Autodesk Inventor part; units mm, degrees
ref_plane "YZ Plane" through (0, 0, 0) normal (1, 0, 0) x (0, 1, 0)
ref_plane "XZ Plane" through (0, 0, 0) normal (0, 1, 0) x (-1, 0, 0)
ref_plane "XY Plane" through (0, 0, 0) normal (0, 0, 1) x (1, 0, 0)
sketch "Boceto1" plane through (0, 0, 0) normal (0, 1, 0) x (-1, 0, 0)
  line L0 (0, 0) -> (0, -8.25)
  line L1 (0, -8.25) -> (3, -8.25)
  line L2 (3, -8.25) -> (3, -16.5)
  line L3 (3, -16.5) -> (0, -16.5)
  line L4 (0, -16.5) -> (0, -24.75)
  line L5 (0, -24.75) -> (3, -24.75)
  line L6 (3, -24.75) -> (3, -33)
  line L7 (3, -33) -> (20, -33)
  line L8 (20, 0) -> (0, 0)
  line L9 (20, -28) -> (8, -28)
  line L10 (8, -28) -> (8, -5)
  line L11 (8, -5) -> (20, -5)
  line L12 (20, -33) -> (20, -28)
  line L13 (20, -5) -> (20, 0)
  dimension "d0" = 8.25
  dimension "d1" = 3
  dimension "d3" = 8.25
extrude "Extrusión1" add sketch "Boceto1" along normal blind 3
sketch "Boceto2" plane through (0, 0, 0) normal (0, -1, 0) x (1, 0, 0)
  line L0 (-8, -28) -> (-8, -5)
  line L1 (-8, -5) -> (-8, -28)
  line L2 (-8, -28) -> (-6, -28)
  line L3 (-6, -28) -> (-6, -5)
  line L4 (-6, -5) -> (-8, -5)
  line L5 (-20, 0) -> (-20, -5)
  line L6 (-20, -5) -> (-18, -5)
  line L7 (-18, -5) -> (-18, 0)
  line L8 (-18, 0) -> (-20, 0)
  line L9 (-20, -33) -> (-20, -28)
  line L10 (-20, -28) -> (-18, -28)
  line L11 (-18, -28) -> (-18, -33)
  line L12 (-18, -33) -> (-20, -33)
extrude "Extrusión2" cut sketch "Boceto2" against normal blind 10
sketch "Boceto5" plane through (0, 0, 0) normal (0, -1, 0) x (1, 0, 0)
  line L0 (-18, -5) -> (-6, -5)
  line L1 (-18, -5) -> (-18, -4.832)
  line L2 (-18, -5) -> (-18, 0)
  line L3 (-18, -4.832) -> (-6, -4.832)
  line L4 (-6, -5) -> (-6, -28)
  line L5 (-6, -4.832) -> (-6, -5)
  line L6 (-6, -5) -> (-18, -5)
  point P0 (0, 0)
  dimension "d22" = 0.168
extrude "Extrusión4" cut sketch "Boceto5" against normal blind 3
properties part number "muñeca7"
Work out the finished part from the listing and answer in its coordinate system (mm). A direction names the side the tool comes from. Give positions to 0.01 mm unless a question says otherwise; leave off trailing zeros. Loops run counter-clockwise (first coordinate to the right, second up) from the corner with the lowest first, then second, coordinate; pieces in that order, holes last. Notation, with made-up numbers: (38.5, 27.5) - (78.5, 27.5) arc R13 cw to (78.5, 39.5) - close; hole circle Ø7 at (32, -16). An arc over 180 degrees is marked (long way). Use CSV: the item, a comma, the result in double quotes. Start each with the question number.
(1) Each of these flat-tipped pins is pushed along its axis until it touches: pin 1 (1.5 mm diameter, centred on x = -2, y = 1.5, fed in from -Z); pin 2 (0.9 mm diameter, centred on y = 1, z = -10.5, fed in from +X). Where does it stop, or does it pass through?
(2) Find section A-A, the plane x = -15.25. Determine the outline of the cut face in (y, z), plus the area to 3 significant figures.
(3) Find section C-C, the plane z = -24. Determine the outline of the cut face in (x, y).
(4) Find section D-D, the plane z = -27.5. Determine the outline of the cut face in (x, y).
(5) A tool of negligible diameter and unlimited length cuts with its end or side. For faces 4 (the face through (-9, 1, 0)), 5 (the face through (-10, 1, -33)), 6 (the face through (-1, 1, -8.25)), 7 (the face through (-3, 1, -29)), 8 (the face through (-12, 1, -28)), from which of +Z, -Z, +X, -X, +Y, -Y can it reach the whole face along a straight path? Write none if from no direction.
(6) Find section B-B, the plane y = 1.85. Determine the outline of the cut face in (x, z), plus the area to 3 significant figures.
(7) Find the intervals of material crossed by L1, parallel to Z at x = -10.5, y = 1; L2, parallel to Z at x = -2, y = 2.3; L3, parallel to X at y = 2.5, z = -27.5, in increasing order.
(8) Determine the mould class of faces 1 (the face through (-5.6, 3, -16.4)), 2 (the face through (-1, 1, -24.75)), 3 (the face through (-3, 1, -12)) for opening direction Z: released by +Z, released by -Z, zero draft, split by the parting line, or undercut.
Results found:
1,pin 1,"z = -24.75"
1,pin 2,"x = -3"
2,outline,"(0, -33) - (3, -33) - (3, -28) - (0, -28) - close; (0, -4.83) - (3, -4.83) - (3, 0) - (0, 0) - close"
2,area,"29.5 mm^2"
3,outline,"(-6, 0) - (0, 0) - (0, 3) - (-6, 3) - close"
4,outline,"(-6, 0) - (-3, 0) - (-3, 3) - (-6, 3) - close"
5,face 4,"+Z, +X, -X, +Y, -Y"
5,face 5,"-Z, +X, -X, +Y, -Y"
5,face 6,"+X, +Y, -Y"
5,face 7,"-Z, +X, +Y, -Y"
5,face 8,"-X, +Y, -Y"
6,outline,"(-18, -33) - (-3, -33) - (-3, -24.75) - (0, -24.75) - (0, -16.5) - (-3, -16.5) - (-3, -8.25) - (0, -8.25) - (0, 0) - (-18, 0) - (-18, -4.83) - (-6, -4.83) - (-6, -28) - (-18, -28) - close"
6,area,"266 mm^2"
7,L1,"-33 to -28, -4.83 to 0"
7,L2,"-24.75 to -16.5, -8.25 to 0"
7,L3,"-6 to -3"
8,face 1,"zero draft"
8,face 2,"released by -Z"
8,face 3,"undercut"
